Can you work these out from the model? Positions are in its coordinate system, mm. Give positions to 0.01 mm unless a question says otherwise; leave off trailing zeros. Order: outer loops, then holes, each group sorted by start corner. A loop starts at its lowest first (then second) coordinate and runs counter-clockwise, first axis right, second up. Notation, with made-up numbers: (52, -26.5) - (108, -26.5) arc R33 cw to (108, 5.5) - close; hole circle Ø3 at (-26.5, 41.5). An arc over 180 degrees is marked (long way). Use one line per item in the form item = value. Start each with the question number.
1) Suppose I cut it at B-B, the plane x = 27.5. Write out the boundary of the cut face in (y, z).
2) Suppose I cut it at A-A, the plane z = -56. Write out the boundary of the cut face in (x, y), and give its area (3 significant figures).
3) Please list where these lines run through material, in increasing order: probe 1 along X at (y, z) = (1.45, -56); probe 2 along Z at (x, y) = (27.5, 1.4).
```python
from build123d import *

# Parameters (mm, degrees)
ESQUISSE1_W             = 80
ESQUISSE1_H             = 80
BOSS_EXTRU_1_DEPTH      = 2
ENL_V_MAT_EXTRU_1_REACH = 4
ESQUISSE2_R             = 1.75


with BuildPart() as part:
    # Esquisse1 → Boss.-Extru.1 (new body)
    with BuildSketch(Plane(origin=(0, 0, 0), x_dir=(1, 0, 0), z_dir=(0, 1, 0))):
        with Locations((40, 40)):
            Rectangle(ESQUISSE1_W, ESQUISSE1_H)
    extrude(amount=BOSS_EXTRU_1_DEPTH)

    # Esquisse2 → Enlèv. mat.-Extru.1 (cut, up to next)
    with BuildSketch(Plane(origin=(0, 2, 0), x_dir=(1, 0, 0), z_dir=(0, 1, 0)), mode=Mode.PRIVATE) as enl_v_mat_extru_1_sk1:
        with Locations((27.5, 56)):
            Circle(ESQUISSE2_R)
    enl_v_mat_extru_1_tool1 = extrude(enl_v_mat_extru_1_sk1.sketch, amount=-ENL_V_MAT_EXTRU_1_REACH, mode=Mode.PRIVATE) & part.part
    add(enl_v_mat_extru_1_tool1.solids().sort_by_distance((27.5, 2, -56))[0], mode=Mode.SUBTRACT)
    # Esquisse2 → Enlèv. mat.-Extru.1 (cut, up to next)
    with BuildSketch(Plane(origin=(0, 2, 0), x_dir=(1, 0, 0), z_dir=(0, 1, 0)), mode=Mode.PRIVATE) as enl_v_mat_extru_1_sk2:
        with Locations((52.5, 56)):
            Circle(ESQUISSE2_R)
    enl_v_mat_extru_1_tool2 = extrude(enl_v_mat_extru_1_sk2.sketch, amount=-ENL_V_MAT_EXTRU_1_REACH, mode=Mode.PRIVATE) & part.part
    add(enl_v_mat_extru_1_tool2.solids().sort_by_distance((52.5, 2, -56))[0], mode=Mode.SUBTRACT)


solid = part.part
```
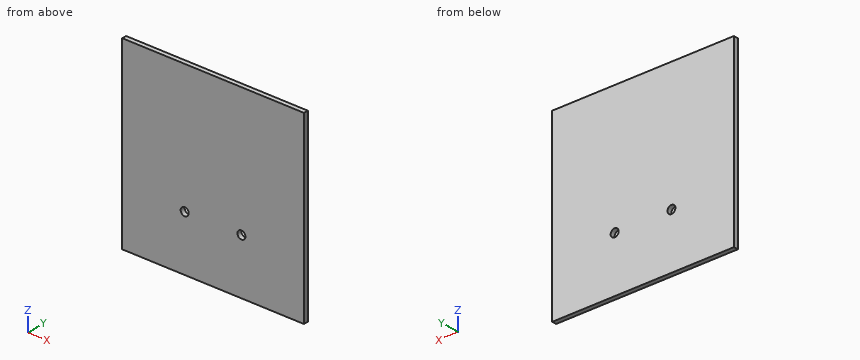
Result sheet:
q1.outline = (0, -80) - (2, -80) - (2, -57.75) - (0, -57.75) - close; (0, -54.25) - (2, -54.25) - (2, 0) - (0, 0) - close
q2.outline = (0, 0) - (25.75, 0) - (25.75, 2) - (0, 2) - close; (29.25, 0) - (50.75, 0) - (50.75, 2) - (29.25, 2) - close; (54.25, 0) - (80, 0) - (80, 2) - (54.25, 2) - close
q2.area = 146 mm²
q3.probe_1 = 0 to 25.75, 29.25 to 50.75, 54.25 to 80
q3.probe_2 = -80 to -57.75, -54.25 to 0
